The drawing under review shows one solid part. Ordinate dimensions are in mm from its lowest x, y, z. A direction names the side the tool comes from. Coordinates: 2 decimals unless noted, no trailing zeros. Write each loop counter-clockwise with the first axis right and the second up, starting at its lowest first coordinate (ties: lowest second). Pieces come first, ordered by that corner, then holes. Notation, with made-up numbers: (-4.75, 15) -> (29.25, 15) arc R15 ccw to (29.25, 30) -> close; hole circle Ø1 at (61.5, 19.5). An arc over 180 degrees is marked (long way). Put each result on its own line as item: value. Start each with the question number.
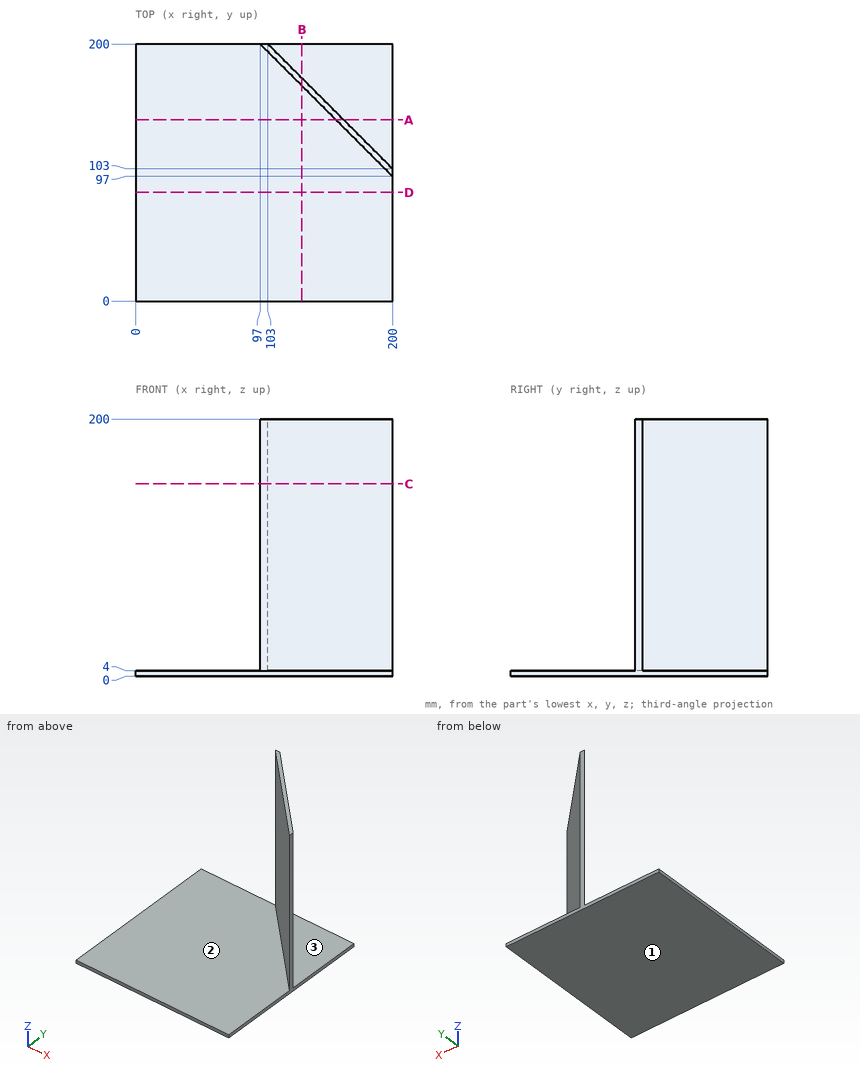
1. Tool access review of the marked faces 1, 2 and 3: name each direction out of +Z, -Z, +X, -X, +Y, -Y from which nothing blocks a thin tool from reaching the whole face with its end or side.
2. Consider section D-D on y = 84.5. State the section outline as (x, z) points.
3. Consider section A-A on y = 141. State the section outline as (x, z) points, then the cut area to 3 significant figures.
4. Consider section B-B on x = 129.5. State the section outline as (y, z) points.
5. Wall thickness on line 1 (Z direction, x = 136, y = 40); line 2 (Y direction, x = 134, z = 28); line 3 (X direction, y = 169.5, z = 58): over which ranges is each line inside the solid? List them lowest first. Write a range as from..to.
6. Insertion check: P1, Ø2, axis at x = 95.5, y = 150, coming from the +Z side; P2, Ø5, axis at y = 124, z = 159.5, coming from the -X side; P3, Ø2, axis at y = 144.5, z = 127.5, coming from the +X side. Each pin has a flat end and moves straight along its axis. Give the tip position at first contact, or say it passes through.
7. Consider section C-C on z = 149.5. State the section outline as (x, y) points, then the cut area to 3 significant figures.
Output values:
1. face 1: -Z, +X, -X, +Y, -Y
1. face 2: +Z, -X, -Y
1. face 3: +Z, +X, +Y
2. outline: (0, 0) -> (200, 0) -> (200, 4) -> (0, 4) -> close
3. outline: (0, 0) -> (200, 0) -> (200, 4) -> (162, 4) -> (162, 200) -> (156, 200) -> (156, 4) -> (0, 4) -> close
3. area: 1,980 mm^2
4. outline: (0, 0) -> (200, 0) -> (200, 4) -> (173.5, 4) -> (173.5, 200) -> (167.5, 200) -> (167.5, 4) -> (0, 4) -> close
5. line 1: z = 0..4
5. line 2: y = 163..169
5. line 3: x = 127.5..133.5
6. P1: stops at z = 4
6. P2: stops at x = 170.5
6. P3: stops at x = 159.5
7. outline: (97, 200) -> (200, 97) -> (200, 103) -> (103, 200) -> close
7. area: 600 mm^2
